Design review of the part built by this model. Coordinates are the model's own, in mm. A direction names the side the tool comes from. Coordinates: 2 decimals unless noted, no trailing zeros. Loops run counter-clockwise (first coordinate to the right, second up) from the corner with the lowest first, then second, coordinate; pieces in that order, holes last. Notation, with made-up numbers: M 83,82 L 128,82 A19 ccw 128,112 Z; hole C 34.5,6 d5. An arc over 180 degrees is marked long. Put each result on its own line as item: value. Start each with the question number.
(1) Take a section at A-A, the plane z = 0. Give the boundary of the cut face in (x, y), then the cut area to 3 significant figures.
(2) Take a section at B-B, the plane z = -16. Give the boundary of the cut face in (x, y) (3 decimals).
(3) For probe 1 along Z at (x, y) = (-15.5, 2); probe 2 along Z at (x, y) = (0, 3.95); probe 3 along Y at (x, z) = (6.3, 17.9), list the stretches that pass through material, from the lowest coordinate up. Write a range as [from, to].
(4) Take a section at C-C, the plane x = 12.5. Give the boundary of the cut face in (y, z).
(5) For faces 4 (the cylindrical face through (5.929, 14.326, 18.535)), 5 (the flat face through (-13, 5, 0)), 6 (the flat face through (21, 2, 0)), 7 (the flat face through (11, 10, -16)), 8 (the flat face through (9.649, 9.93, -9.413)), list the 3-axis set-ups (+Z, -Z, +X, -X, +Y, -Y) from which the entire face can be reached by the end or side of a thin tool; tool diameter is ignored.
(6) Take a section at D-D, the plane x = 6.3. Give the boundary of the cut face in (y, z) (3 decimals), then the cut area to 3 significant figures.
(7) Clearance check with flat-ended pins moving along their axes: pin 1 (4 mm diameter, centred on x = -7, z = -5, fed in from -Y); pin 2 (4.5 mm diameter, centred on y = 9.5, z = -15, fed in from -X); pin 3 (9 mm diameter, centred on x = 5, z = -14.5, fed in from +Y); pin 4 (3.5 mm diameter, centred on y = 12.5, z = 14, fed in from +X). State where each tip first meets the part, or that it passes through.
(8) The part is to be moulded in two halves that separate along Y. For faces 1 (the cylindrical face through (7.385, 11.05, -15.112)), 2 (the cylindrical face through (-14.601, 2.535, -16.845)), 3 (the flat face through (6, 15, -16)), say which applies: +Y half, -Y half, draft (parallel to the pull), parting line (faces both ways), or undercut.
```python
from build123d import *

# Parameters (mm, degrees)
SKETCH1_W           = 42
SKETCH1_H           = 42
SKETCH1_R           = 12
BOSS_EXTRUDE1_DEPTH = 5
SKETCH2_R           = 1.625
CUT_EXTRUDE1_DEPTH  = 8
BOSS_EXTRUDE2_DEPTH = 10
SKETCH4_R           = 1.175
CUT_EXTRUDE2_DEPTH  = 42
SKETCH5_R           = 5
CUT_EXTRUDE3_DEPTH  = 10
SKETCH6_R           = 2.85
CUT_EXTRUDE4_DEPTH  = 5
BOSS_EXTRUDE3_DEPTH = 1


with BuildPart() as part:
    # Sketch1 → Boss-Extrude1 (new body)
    with BuildSketch(Plane(origin=(0, 0, 0), x_dir=(1, 0, 0), z_dir=(0, 1, 0))):
        Rectangle(SKETCH1_W, SKETCH1_H)
        Circle(SKETCH1_R, mode=Mode.SUBTRACT)
    extrude(amount=BOSS_EXTRUDE1_DEPTH)

    # Sketch2 → Cut-Extrude1 (cut)
    with BuildSketch(Plane(origin=(0, 5, 0), x_dir=(1, 0, 0), z_dir=(0, 1, 0))):
        with Locations((-15.475, 15.475)):
            Circle(SKETCH2_R)
        with Locations((15.475, 15.475)):
            Circle(SKETCH2_R)
        with Locations((15.475, -15.475)):
            Circle(SKETCH2_R)
        with Locations((-15.475, -15.475)):
            Circle(SKETCH2_R)
    extrude(amount=-CUT_EXTRUDE1_DEPTH, mode=Mode.SUBTRACT)

    # Sketch3 → Boss-Extrude2 (add)
    with BuildSketch(Plane(origin=(0, 5, 0), x_dir=(1, 0, 0), z_dir=(0, 1, 0))):
        with BuildLine():
            Line((0, 12), (0, 21))
            Line((0, 21), (11, 21))
            Line((11, 21), (11, 10.102949137))
            Line((11, 10.102949137), (8.260404548, 8.704350447))
            ThreePointArc((8.260404548, 8.704350447), (4.446785054, 11.145676412), (0, 12))
        make_face()
        with BuildLine():
            Line((0, -21), (11, -21))
            Line((11, -21), (11, -10.102949137))
            Line((11, -10.102949137), (8.260404548, -8.704350447))
            ThreePointArc((8.260404548, -8.704350447), (4.446785054, -11.145676412), (0, -12))
            Line((0, -12), (0, -21))
        make_face()
    extrude(amount=BOSS_EXTRUDE2_DEPTH)

    # Sketch4 → Cut-Extrude2 (cut)
    with BuildSketch(Plane.XY.offset(21)):
        with Locations((6.3, 11.5)):
            Circle(SKETCH4_R)
    extrude(amount=-CUT_EXTRUDE2_DEPTH, mode=Mode.SUBTRACT)

    # Sketch5 → Cut-Extrude3 (cut)
    with BuildSketch(Plane(origin=(0, 5, 0), x_dir=(1, 0, 0), z_dir=(0, 1, 0))):
        with Locations((12.5, 0)):
            Circle(SKETCH5_R)
    extrude(amount=-CUT_EXTRUDE3_DEPTH, mode=Mode.SUBTRACT)

    # Sketch6 → Cut-Extrude4 (cut)
    with BuildSketch(Plane.XY.offset(21)):
        with Locations((6.3, 11.5)):
            Circle(SKETCH6_R)
    extrude(amount=-CUT_EXTRUDE4_DEPTH, mode=Mode.SUBTRACT)

    # Sketch7 → Boss-Extrude3 (add)
    with BuildSketch(Plane(origin=(0, 15, 0), x_dir=(1, 0, 0), z_dir=(0, 1, 0))):
        with BuildLine():
            Line((0, -21), (11, -21))
            Line((11, -21), (11, -10.102949137))
            Line((11, -10.102949137), (8.260404548, -8.704350447))
            ThreePointArc((8.260404548, -8.704350447), (4.446785054, -11.145676412), (0, -12))
            Line((0, -12), (0, -21))
        make_face()
    extrude(amount=BOSS_EXTRUDE3_DEPTH)


solid = part.part
```
Computed values:
1. outline: M -21,0 L -12,0 L -12,5 L -21,5 Z; M 17.5,0 L 21,0 L 21,5 L 17.5,5 Z
1. area: 62.5 mm^2
2. outline: M -21,0 L -17.013,0 L -17.013,5 L -21,5 Z; M -13.937,0 L 13.937,0 L 13.937,5 L 11,5 L 11,15 L 0,15 L 0,5 L -13.937,5 Z; M 17.013,0 L 21,0 L 21,5 L 17.013,5 Z; hole C 6.3,11.5 d2.35
3. probe 1: z = [-21, -17.1], [-13.85, 13.85], [17.1, 21]
3. probe 2: z = [-21, -12], [12, 21]
3. probe 3: y = [0, 8.65], [14.35, 16]
4. outline: M 0,-21 L 5,-21 L 5,-5 L 0,-5 Z; M 0,5 L 5,5 L 5,21 L 0,21 Z
5. face 4: +Z
5. face 5: +Z, -Z, -X, +Y
5. face 6: +Z, -Z, +X, +Y, -Y
5. face 7: +Z, -Z, +X, +Y
5. face 8: +X, +Y
6. outline: M 0,-21 L 10.325,-21 L 10.325,-10.213 L 0,-10.213 Z; M 0,10.213 L 10.325,10.213 L 10.325,16 L 8.65,16 L 8.65,21 L 0,21 Z; M 12.675,-21 L 15,-21 L 15,-10.213 L 12.675,-10.213 Z; M 12.675,10.213 L 16,10.213 L 16,21 L 14.35,21 L 14.35,16 L 12.675,16 Z
6. area: 267 mm^2
7. pin 1: passes through
7. pin 2: stops at x = 0
7. pin 3: stops at y = 15
7. pin 4: stops at x = 11
8. face 1: undercut
8. face 2: draft
8. face 3: +Y half
